Source: CAD feature listing. Evaluate the final solid. Frame: model axes, mm. A direction names the side the tool comes from. Round coordinates to 2 decimals unless told otherwise and drop trailing zeros. Order: outer loops, then holes, each group sorted by start corner. A loop starts at its lowest first (then second) coordinate and runs counter-clockwise, first axis right, second up. Notation, with made-up numbers: (42, 31) -> (49, 31) arc R28 cw to (49, 63) -> close; hole circle Ø11 at (56, 87.25). An arc over 180 degrees is marked (long way). One line per item, written item: value. Start each with the question number.
1) Pin query (flat end, axial travel): P1, Ø9, axis at x = 56, y = 9, coming from the -Z side; P2, Ø4, axis at y = 10, z = 56.21, coming from the +X side; P3, Ø1, axis at x = -20, y = 12, coming from the +Z side; P4, Ø2.5, axis at y = 17.5, z = 48.71, coming from the +X side. Return the tip coordinate at first contact, or that it passes through.
2) Section A-A (x = -56). Return the cut outline in (y, z).
3) Mould query, pull axis Z, two halves, no side actions, for faces 1 (the face through (18.236, 17.148, 55.207)), 2 (the face through (1, 15, -81.785)), 3 (the face through (-1, 15, -83.785)), 4 (the face through (98, 13, -32)). Classes: pulls with the +Z half, pulls with the -Z half, needs draft (parallel to the pull), parting line crosses it, or undercut.
4) Ray query, L1, parallel to X at y = 12.5, z = 8; L2, parallel to Z at x = 80.5, y = 12.75; L3, parallel to Z at x = -79, y = 7. Return the intervals inside material, ascending.
5) Section B-B (z = 32). Return the cut outline in (x, y).
6) Reachability of faces 5 (the face through (-98, 13, -33)), 6 (the face through (33.75, 10, 38)), 7 (the face through (31.75, 10, 38)), 8 (the face through (-42, 11, 18.215)) from +Z, -Z, +X, -X, +Y, -Y: full face, straight path, thin tool, end or side. Return the list, or none.
```python
from build123d import *

# Parameters (mm, degrees)
EXTRUDE_1_DEPTH          = 20
CUT_EXTRUDE_1_DEPTH      = 160.088219443
CUT_EXTRUDE_1_DEPTH_BACK = 160.088219443
SKETCH_6_R               = 5
SKETCH_6_3_R             = 1.5
CUT_EXTRUDE_2_DEPTH      = 160.088219443
PATTERN_CIRCULAR_1_COUNT = 4
FILLET_1_R               = 10
CUT_EXTRUDE_3_DEPTH      = 218.761335102
CUT_EXTRUDE_3_DEPTH_BACK = 218.761335102
EXTRUDE_START            = -98
EXTRUDE_2_DEPTH          = 117.25
EXTRUDE_START_2          = 31.75
EXTRUDE_2_2_DEPTH        = 66.25
EXTRUDE_START_3          = 17.25
EXTRUDE_2_3_DEPTH        = 2
EXTRUDE_2_4_DEPTH        = 2
CUT_EXTRUDE_4_DEPTH      = 132.984844075
CUT_EXTRUDE_4_DEPTH_BACK = 132.984844075
SKETCH_12_W              = 119.060862832
SKETCH_12_H              = 18
SKETCH_12_W_2            = 69.668977306


# Read off the part's stored shape, not the designer's step: 凸台-拉伸2
with BuildPart() as part:
    # 草图2 → 凸台-拉伸1 (new body)
    with BuildSketch(Plane(origin=(0, 0, 0), x_dir=(1, 0, 0), z_dir=(0, 1, 0))):
        Polygon((17.25, -36.214565314), (-100, -36.214565314), (-100, 83.785434686), (100, 83.785434686), (100, -36.214565314), (33.75, -36.214565314), (33.75, -58.214565314), (31.75, -58.214565314), (31.75, -34.214565314), (98, -34.214565314), (98, 81.785434686), (-98, 81.785434686), (-98, -34.214565314), (19.25, -34.214565314), (19.25, -58.214565314), (17.25, -58.214565314), align=None)
    extrude(amount=EXTRUDE_1_DEPTH)

    # 草图6 → 切除-拉伸1 (cut, two sides: drawn at the far end of the back side and taken through both)
    with BuildSketch(Plane(origin=(33.75, 0, 0), x_dir=(0, 0, -1), z_dir=(1, 0, 0)).offset(-CUT_EXTRUDE_1_DEPTH_BACK)):
        with Locations((-48.714565314, 10)):
            Circle(SKETCH_6_R)
    extrude(amount=CUT_EXTRUDE_1_DEPTH + CUT_EXTRUDE_1_DEPTH_BACK, mode=Mode.SUBTRACT)

    # 草图6<3> → 切除-拉伸2 (cut, symmetric)
    with BuildSketch(Plane(origin=(33.75, 0, 0), x_dir=(0, 0, -1), z_dir=(1, 0, 0))):
        with Locations((-48.714565314, 17.5)):
            Circle(SKETCH_6_3_R)
    cut_extrude_2 = extrude(amount=CUT_EXTRUDE_2_DEPTH, both=True, mode=Mode.SUBTRACT)

    # 阵列(圆周)1: 切除-拉伸2 ×4 about axis
    pattern_circular_1_axis = Axis((0, 10, 48.714565314), (1, 0, 0))
    for i in range(1, PATTERN_CIRCULAR_1_COUNT):
        add(cut_extrude_2.rotate(pattern_circular_1_axis, i * 360 / PATTERN_CIRCULAR_1_COUNT), mode=Mode.SUBTRACT)

    # 圆角1
    fillet_1_edges = [part.edges().sort_by_distance(p)[0] for p in [
        (32.75, 20, 58.214565314),
        (32.75, 0, 58.214565314),
        (18.25, 0, 58.214565314),
        (18.25, 20, 58.214565314),
    ]]
    fillet(fillet_1_edges, radius=FILLET_1_R - 0.0001)  # a hair under: the kernel refuses the full size

    # 草图8 → 切除-拉伸3 (cut, two sides: drawn at the far end of the back side and taken through both)
    with BuildSketch(Plane.ZY.offset(100).offset(-CUT_EXTRUDE_3_DEPTH_BACK)):
        Polygon((41.803939726, 0), (-83.785434686, 10), (-83.785434686, 0), align=None)
    extrude(amount=CUT_EXTRUDE_3_DEPTH + CUT_EXTRUDE_3_DEPTH_BACK, mode=Mode.SUBTRACT)

    # 凸台-拉伸2 outline → 凸台-拉伸2 (add)
    with BuildSketch(Plane.YZ.offset(EXTRUDE_START)):
        Polygon((20, 16.214565314), (20, 18.214565314), (1.878293807, 18.214565314), (2.037542948, 16.214565314), align=None)
    extrude(amount=EXTRUDE_2_DEPTH)

    # Extrude 2 2 outline → Extrude 2 2 (add)
    with BuildSketch(Plane.YZ.offset(EXTRUDE_START_2)):
        Polygon((20, 16.214565314), (20, 18.214565314), (1.878293807, 18.214565314), (2.037542948, 16.214565314), align=None)
    extrude(amount=EXTRUDE_2_2_DEPTH)

    # Extrude 2 3 outline → Extrude 2 3 (add)
    with BuildSketch(Plane.YZ.offset(EXTRUDE_START_3)):
        Polygon((20, 18.214565314), (20, 34.214565314), (0.604300678, 34.214565314), (1.878293807, 18.214565314), align=None)
    extrude(amount=EXTRUDE_2_3_DEPTH)

    # Extrude 2 4 outline → Extrude 2 4 (add)
    with BuildSketch(Plane.YZ.offset(EXTRUDE_START_2)):
        Polygon((20, 18.214565314), (20, 34.214565314), (0.604300678, 34.214565314), (1.878293807, 18.214565314), align=None)
    extrude(amount=EXTRUDE_2_4_DEPTH)

    # 草图12 → 切除-拉伸4 (cut, two sides: drawn at the far end of the back side and taken through both)
    with BuildSketch(Plane(origin=(0, 0, 0), x_dir=(1, 0, 0), z_dir=(0, 1, 0)).offset(-CUT_EXTRUDE_4_DEPTH_BACK)):
        with Locations((-42.280431416, -27.214565314)):
            Rectangle(SKETCH_12_W, SKETCH_12_H)
        with Locations((68.584488653, -27.214565314)):
            Rectangle(SKETCH_12_W_2, SKETCH_12_H)
    extrude(amount=CUT_EXTRUDE_4_DEPTH + CUT_EXTRUDE_4_DEPTH_BACK, mode=Mode.SUBTRACT)


solid = part.part
```
Findings:
1. P1: z = -83.79
1. P2: x = 33.75
1. P3: z = 18.21
1. P4: through
2. outline: (1.88, 18.21) -> (2.04, 16.21) -> (20, 16.21) -> (20, 18.21) -> close; (9.84, -81.79) -> (10, -83.79) -> (20, -83.79) -> (20, -81.79) -> close
3. face 1: pulls with the +Z half
3. face 2: undercut
3. face 3: pulls with the -Z half
3. face 4: undercut
4. L1: -100 to -98, 98 to 100
4. L2: -83.79 to -81.79, 16.21 to 18.21
4. L3: 16.21 to 18.21
5. outline: (17.25, 0.78) -> (19.25, 0.78) -> (19.25, 20) -> (17.25, 20) -> close; (31.75, 0.78) -> (33.75, 0.78) -> (33.75, 20) -> (31.75, 20) -> close
6. face 5: +Y, -Y
6. face 6: +Z, +X, +Y, -Y
6. face 7: +Z, +Y, -Y
6. face 8: +Z, -X, +Y, -Y
